Verification items for this drawing (mm, ordinates from the low corner). A direction names the side the tool comes from. Round coordinates to 2 decimals unless told otherwise and drop trailing zeros. Loops run counter-clockwise (first coordinate to the right, second up) from the corner with the lowest first, then second, coordinate; pieces in that order, holes last. Notation, with made-up numbers: (-7.5, 79.5) - (51.5, 79.5) arc R24 cw to (51.5, 93.5) - close; hole circle Ø10 at (19, 75.5). An arc over 180 degrees is marked (long way). Write item = value, one per line.
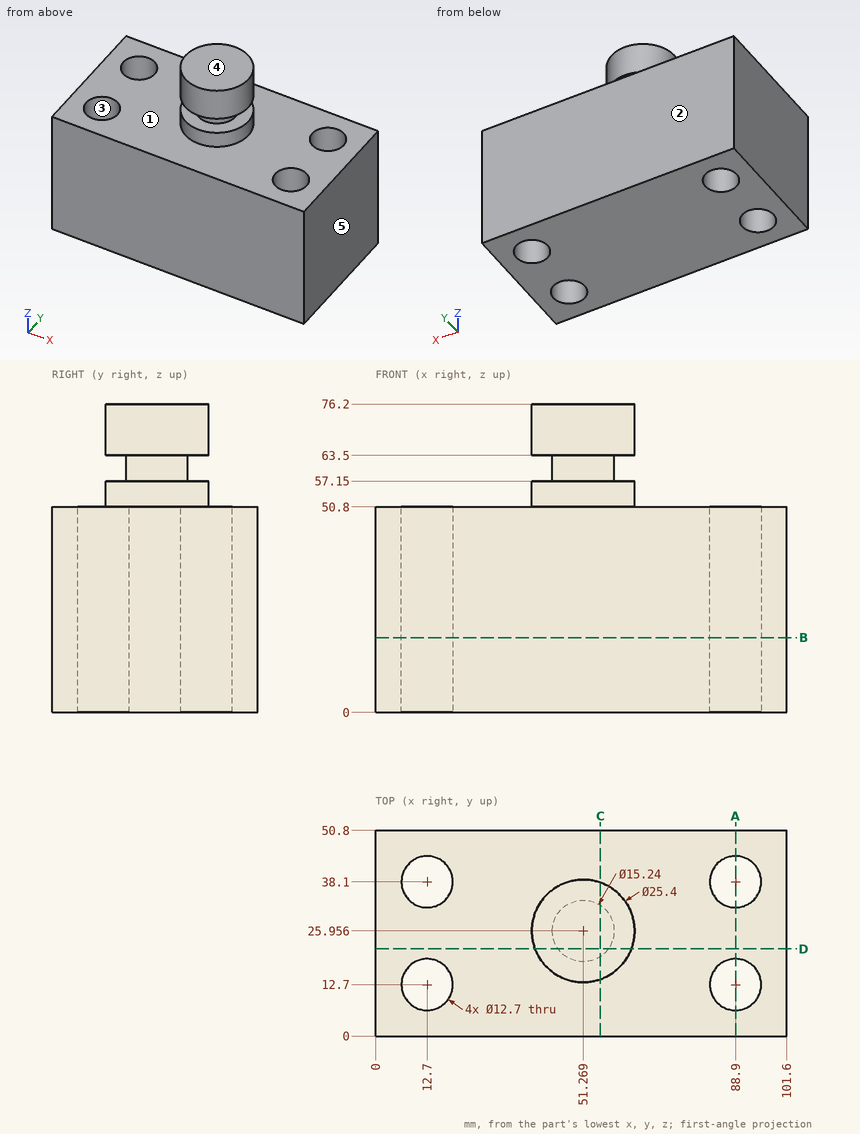
(1) Section check A-A (x = 88.9). Enter the section's corners in (y, z), then the cut area to 3 significant figures.
Answers follow:
outline = (0, 0) - (6.35, 0) - (6.35, 50.8) - (0, 50.8) - close; (19.05, 0) - (31.75, 0) - (31.75, 50.8) - (19.05, 50.8) - close; (44.45, 0) - (50.8, 0) - (50.8, 50.8) - (44.45, 50.8) - close
area = 1,290 mm²
(2) Set-up check for the marked faces 1 and 2: record each of +Z, -Z, +X, -X, +Y, -Y from which the full face is reachable in a straight line by a thin tool's end or side.
Answers follow:
face_1 = +Z
face_2 = +Z, -Z, +X, -X, +Y
(3) Section check C-C (x = 55.5). Enter the section's corners in (y, z).
Answers follow:
outline = (0, 0) - (50.8, 0) - (50.8, 50.8) - (37.93, 50.8) - (37.93, 57.15) - (32.29, 57.15) - (32.29, 63.5) - (37.93, 63.5) - (37.93, 76.2) - (13.98, 76.2) - (13.98, 63.5) - (19.62, 63.5) - (19.62, 57.15) - (13.98, 57.15) - (13.98, 50.8) - (0, 50.8) - close
(4) Scan lines: L1, parallel to Y at x = 12.7, z = 36.5; L2, parallel to Z at x = 56, y = 32; L3, parallel to X at y = 12, z = 13. Record each from-to range of solid material in increasing order. Write a range as [from, to].
Answers follow:
L1 = [0, 6.35], [19.05, 31.75], [44.45, 50.8]
L2 = [0, 57.15], [63.5, 76.2]
L3 = [0, 6.39], [19.01, 82.59], [95.21, 101.6]
(5) Gauge pin test, flat ends, axial feed: pin 1 (4 mm diameter, centred on x = 51, z = 62.5, fed in from +Y); pin 2 (7.5 mm diameter, centred on x = 88.9, y = 12.7, fed in from +Z); pin 3 (16.5 mm diameter, centred on x = 12.7, y = 12.7, fed in from +Z). Record the tip position at first contact, or that the pin passes through.
Answers follow:
pin_1 = 38.66
pin_2 = through
pin_3 = 50.8
(6) Mould release check, pull along X, two halves, no side actions. Record for the marked faces 3, 4 and 5: pulls with the +X half, pulls with the -X half, needs draft (parallel to the pull), parting line crosses it, or undercut.
Answers follow:
face_3 = undercut
face_4 = needs draft
face_5 = pulls with the +X half
(7) Section check B-B (z = 18.5). Enter the section's corners in (x, y).
Answers follow:
outline = (0, 0) - (101.6, 0) - (101.6, 50.8) - (0, 50.8) - close; hole circle Ø12.7 at (12.7, 12.7); hole circle Ø12.7 at (12.7, 38.1); hole circle Ø12.7 at (88.9, 12.7); hole circle Ø12.7 at (88.9, 38.1)
(8) Section check D-D (y = 21.5). Enter the section's corners in (x, z), then the cut area to 3 significant figures.
Answers follow:
outline = (0, 0) - (101.6, 0) - (101.6, 50.8) - (63.16, 50.8) - (63.16, 57.15) - (57.45, 57.15) - (57.45, 63.5) - (63.16, 63.5) - (63.16, 76.2) - (39.38, 76.2) - (39.38, 63.5) - (45.09, 63.5) - (45.09, 57.15) - (39.38, 57.15) - (39.38, 50.8) - (0, 50.8) - close
area = 5,690 mm²
